Work out the finished part from the listing and answer in its coordinate system (mm). A direction names the side the tool comes from. Round coordinates to 2 decimals unless told otherwise and drop trailing zeros. Loops run counter-clockwise (first coordinate to the right, second up) from the corner with the lowest first, then second, coordinate; pieces in that order, holes last.
```python
from build123d import *

# Parameters (mm, degrees)
FILLET4_R = 0.127


with BuildPart() as part:
    # Sketch1 → Revolve1 (revolve)
    with BuildSketch(Plane.XY, mode=Mode.PRIVATE) as revolve1_sk:
        Polygon((0, 0), (-17.399, 0), (-17.399, 1.5875), (-15.7607, 1.5875), (-15.7607, 3.0099), (-17.399, 3.0099), (-17.399, 12.5349), (-18.9738, 12.5349), (-18.9738, 15.0749), (-17.018, 15.0749), (-17.018, 18.6309), (-18.9738, 18.6309), (-18.9738, 24.9809), (0, 24.9809), align=None)
    revolve(revolve1_sk.sketch.rotate(Axis((0, 0, 0), (0, 1, 0)), 270), axis=Axis((0, 0, 0), (0, 1, 0)))

    # Fillet4
    fillet4_edges = [part.edges().sort_by_distance(p)[0] for p in [
        (0, 18.6309, 17.018),
        (0, 15.0749, 17.018),
    ]]
    fillet(fillet4_edges, radius=FILLET4_R)


solid = part.part
```
1. Consider probe 1 along Y at (x, z) = (14.5, 8.5); probe 2 along X at (y, z) = (12, 0.5); probe 3 along Y at (x, z) = (15.5, -9). Determine where each line is inside the solid, lowest interval first.
Answer key:
probe 1: y = 0 to 1.59, 3.01 to 24.98
probe 2: x = -17.39 to 17.39
probe 3: y = 12.53 to 15.07, 18.63 to 24.98
2. Determine the mould class of faces 1 (the face through (10.587, 7.839, 13.807)), 2 (the face through (6, 12.535, 17)), 3 (the face through (-4.734, 2.309, -15.033)) for opening direction Y: +Y half, -Y half, draft (parallel to the pull), parting line (faces both ways), or undercut.
Answer key:
face 1: draft
face 2: -Y half
face 3: undercut
3. Given pin 1 (2 mm diameter, centred on x = 12, y = 15, fed in from -Z); pin 2 (3 mm diameter, centred on x = 8.5, y = 7, fed in from -Z); pin 3 (4 mm diameter, centred on x = -12, y = 11.5, fed in from +Z), each flat-ended and moving along its own axis, determine where each tip first touches the part or whether it passes through.
Answer key:
pin 1: stops at z = -15.46
pin 2: stops at z = -15.93
pin 3: stops at z = 15.94
4. Find section C-C (y = 8.5). Write down the section's boundary in (x, z).
Answer key:
outline: circle Ø34.8 at (0, 0)
5. Which of the six approach directions +Z, -Z, +X, -X, +Y, -Y give full straight-line access (tool end or side, diameter ignored) to faces 4 (the face through (17, 15.075, 4)), 5 (the face through (10.587, 0.805, 13.807)), 6 (the face through (-18.812, 21.85, 2.47))?
Answer key:
face 4: none
face 5: -Y
face 6: +Y, -Y
6. Find section D-D (y = 23.25). Write down the section's boundary in (x, z).
Answer key:
outline: circle Ø37.95 at (0, 0)
